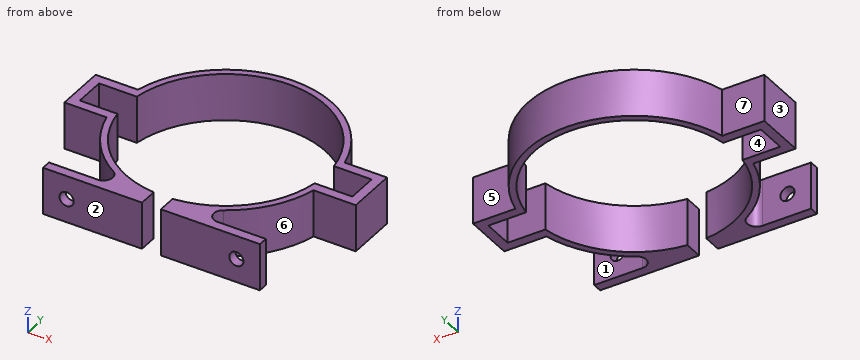
Autodesk Inventor part; units mm, degrees
ref_plane "YZ Plane" through (0, 0, 0) normal (1, 0, 0) x (0, 1, 0)
ref_plane "XZ Plane" through (0, 0, 0) normal (0, 1, 0) x (-1, 0, 0)
ref_plane "XY Plane" through (0, 0, 0) normal (0, 0, 1) x (1, 0, 0)
sketch "Sketch1" plane through (0, 0, 0) normal (0, 0, 1) x (1, 0, 0)
  circle A0 centre (0, 0) radius 21.15 construction
  line L0 (-18, -25) -> (18, -25) construction
  line L1 (-18, -25) -> (-18, -38.1522) construction
  line L2 (18, -25) -> (18, -38.1522) construction
  line L3 (-23, -23) -> (-23, -25)
  line L4 (-23, -25) -> (-2, -25)
  line L5 (-2, -21.0552) -> (-2, -25)
  line L6 (2, -21.0552) -> (2, -25)
  line L7 (2, -25) -> (23, -25)
  line L8 (23, -25) -> (23, -23)
  line L9 (23, -23) -> (12.7162, -23)
  line L10 (-23, -23) -> (-12.7162, -23)
  arc A1 (2, -21.0552) -> (-2, -21.0552) centre (0, 0) ccw
  arc A2 (11.6803, -19.2892) -> (12.7162, -23) centre (12.7162, -21) ccw
  arc A3 (-12.7162, -23) -> (-11.6803, -19.2892) centre (-12.7162, -21) ccw
  arc A4 (-21.9303, -5.25) -> (-11.6803, -19.2892) centre (0, 0) ccw
  arc A5 (11.6803, -19.2892) -> (21.9303, -5.25) centre (0, 0) ccw
  arc A6 (21.9303, 5.25) -> (-21.9303, 5.25) centre (0, 0) ccw
  line L11 (20.8988, 3.25) -> (28.8988, 3.25)
  line L12 (28.8988, 3.25) -> (28.8988, -3.25)
  line L13 (28.8988, -3.25) -> (20.8988, -3.25)
  line L14 (20.8988, -5.25) -> (30.8988, -5.25)
  line L15 (30.8988, -5.25) -> (30.8988, 5.25)
  line L16 (30.8988, 5.25) -> (20.8988, 5.25)
  line L17 (-21.9303, 5.25) -> (-30.8988, 5.25)
  line L18 (-30.8988, 5.25) -> (-30.8988, -5.25)
  line L19 (-30.8988, -5.25) -> (-21.9303, -5.25)
  line L20 (-20.8988, -3.25) -> (-28.8988, -3.25)
  line L21 (-28.8988, -3.25) -> (-28.8988, 3.25)
  line L22 (-28.8988, 3.25) -> (-20.8988, 3.25)
  point P0 (0, -25)
  point P1 (28.8988, 0)
  point P2 (-28.8988, 0)
  dimension "d13" = 42.3
  dimension "d1" = 25
  dimension "d2" = 36
  dimension "d3" = 2
  dimension "d5" = 5
  dimension "d6" = 2
  dimension "d7" = 4
  dimension "d19" = 22.55
  dimension "d20" = 8
  dimension "d21" = 6.5
  dimension "d22" = 2
  dimension "d23" = 6.5
  dimension "d24" = 8
  dimension "d25" = 2
  dimension "d26" = 2
  dimension "d27" = 2
extrude "Extrusion1" add sketch "Sketch1" along normal blind 10 contours L10 A3 A4 L19 L18 L17 A6 L16 L15 L14 A5 A2 L9 L8 L7 L6 A1 L13 L12 L11 L22 L21 L20 L5 L4 L3
sketch "Sketch2" plane through (2, -25, 0) normal (0, -1, 0) x (1, 0, 0)
  circle A0 centre (16, 5) radius 1.5
  line L0 (21, 0) -> (21, 10)
  point P0 (-2, 0)
  point P1 (16, 0)
  point P2 (16, 0)
  point P3 (16, 0)
  point P4 (21, 5)
  dimension "d10" = 3
extrude "Extrusion2" cut sketch "Sketch2" against normal up to surface (2 mm away)
mirror "Mirror1" about plane through (0, 0, 0) normal (1, 0, 0) of "Extrusion2"
properties part number "OmegaRing" material "ABS Plastic"
Can you work these out from the model? Positions are in its coordinate system, mm. Face numbers are marked on the shaded views. A direction names the side the tool comes from. Coordinates: 2 decimals unless noted, no trailing zeros. Loops run counter-clockwise (first coordinate to the right, second up) from the corner with the lowest first, then second, coordinate; pieces in that order, holes last. Notation, with made-up numbers: (40.5, 16) - (89.5, 16) arc R28 ccw to (89.5, 51) - close; hole circle Ø5 at (58, 37.25). An arc over 180 degrees is marked (long way). Answer as a JSON object with one key per item and string values. Group by question number.
Item 1: For pin 1 (2.5 mm diameter, centred on x = 18, z = 5, fed in from -Y); pin 2 (3 mm diameter, centred on x = -18, y = -3, fed in from -Z); pin 3 (3 mm diameter, centred on x = 13, y = 18, fed in from -Z); pin 4 (1 mm diameter, centred on x = -13, z = 1.5, fed in from +Y), each with a flat end and sliding along its axis, tell me the tip position at first contact or that it passes through.
Item 2: If we section it at B-B (x = -3): List the corners of the cut face in (y, z) for me.
Item 3: If we section it at D-D (z = 7.5): List the corners of the cut face in (x, y) for me, plus the area to 3 significant figures.
Item 4: If we section it at A-A (y = -6): List the corners of the cut face in (x, z) for me.
Item 5: On a 3-axis mill with a long thin cutter (end or side, diameter ignored), from which of +Z, -Z, +X, -X, +Y, -Y can I reach the whole of each face in a straight line? I mean the marked faces 4, 5, 6 and 7. Say none if no direction works.
Item 6: If we mould it in two halves opening along Y, with no side actions, what happens to the marked faces 1, 2 and 3? For each: released by +Y, released by -Y, zero draft, split by the parting line, or undercut.
Item 7: If we section it at C-C (x = -18): List the corners of the cut face in (y, z) for me, plus the area to 3 significant figures.
Item 8: If I drill on L1, parallel to Y at x = 22, z = 6; L2, parallel to Y at x = -26, z = 9.5; L3, parallel to Z at x = -18, y = -24, over which ranges is the centre line in solid material (lowest first)? Write a range as from..to.
Returned:
{
 "1": {"pin 1": "stops at y = -15.1", "pin 2": "passes through", "pin 3": "stops at z = 0", "pin 4": "stops at y = 18.77"},
 "2": {"outline": "(-25, 0) - (-20.94, 0) - (-20.94, 10) - (-25, 10) - close; (20.94, 0) - (22.35, 0) - (22.35, 10) - (20.94, 10) - close"},
 "3": {"outline": "(-30.9, -5.25) - (-21.93, -5.25) arc R22.55 ccw to (-11.68, -19.29) arc R2 cw to (-12.72, -23) - (-23, -23) - (-23, -25) - (-2, -25) - (-2, -21.06) arc R21.15 cw to (-20.9, -3.25) - (-28.9, -3.25) - (-28.9, 3.25) - (-20.9, 3.25) arc R21.15 cw to (20.9, 3.25) - (28.9, 3.25) - (28.9, -3.25) - (20.9, -3.25) arc R21.15 cw to (2, -21.06) - (2, -25) - (23, -25) - (23, -23) - (12.72, -23) arc R2 cw to (11.68, -19.29) arc R22.55 ccw to (21.93, -5.25) - (30.9, -5.25) - (30.9, 5.25) - (21.93, 5.25) arc R22.55 ccw to (-21.93, 5.25) - (-30.9, 5.25) - close", "area": "377 mm²"},
 "4": {"outline": "(-21.74, 0) - (-20.28, 0) - (-20.28, 10) - (-21.74, 10) - close; (20.28, 0) - (21.74, 0) - (21.74, 10) - (20.28, 10) - close"},
 "5": {"face 4": "+Z, -Z", "face 5": "+Z, -Z, +X, +Y", "face 6": "+Z, -Z, +X", "face 7": "+Z, -Z, -X, +Y"},
 "6": {"face 1": "undercut", "face 2": "released by -Y", "face 3": "zero draft"},
 "7": {"outline": "(-25, 0) - (-23, 0) - (-23, 3.5) - (-25, 3.5) - close; (-25, 6.5) - (-23, 6.5) - (-23, 10) - (-25, 10) - close; (-13.58, 0) - (-11.11, 0) - (-11.11, 10) - (-13.58, 10) - close; (11.11, 0) - (13.58, 0) - (13.58, 10) - (11.11, 10) - close", "area": "63.6 mm²"},
 "8": {"L1": "y = -25..-23, -5.25..-3.25, 3.25..5.25", "L2": "y = -5.25..-3.25, 3.25..5.25", "L3": "z = 0..3.5, 6.5..10"}
}
